Verification items for the finished model (mm, model axes). Face numbers are marked on the shaded views. A direction names the side the tool comes from. Coordinates: 2 decimals unless noted, no trailing zeros. Write each loop counter-clockwise with the first axis right and the second up, starting at its lowest first coordinate (ties: lowest second). Pieces come first, ordered by that corner, then holes. Notation, with made-up numbers: (84.5, -33.75) -> (118.5, -33.75) arc R22 ccw to (118.5, -25.75) -> close; hole circle Ø8 at (17, 35.5). An arc over 180 degrees is marked (long way). Answer in a Markdown table with one row per item.
```python
from build123d import *

# Parameters (mm, degrees)
SKETCH1_R           = 9
BOSS_EXTRUDE1_DEPTH = 4.8
SKETCH2_R           = 5
BOSS_EXTRUDE2_DEPTH = 3.5
SKETCH3_R           = 2.75
CUT_EXTRUDE1_DEPTH  = 6.8
CHAMFER1_SIZE       = 2
CHAMFER2_SIZE       = 0.6
CHAMFER2_SIZE_2     = 0.889536581
SKETCH4_R           = 1.25
CUT_EXTRUDE2_DEPTH  = 16.081910128
CIRPATTERN1_COUNT   = 7
FILLET1_R           = 1
SKETCH5_R           = 2
CUT_EXTRUDE3_DEPTH  = 16.081910248
CHAMFER3_SIZE       = 0.6
FILLET2_R           = 0.4


with BuildPart() as part:
    # Sketch1 → Boss-Extrude1 (new body)
    with BuildSketch(Plane(origin=(0, 0, 0), x_dir=(1, 0, 0), z_dir=(0, 1, 0))):
        with Locations(Location((0, 0, 0), (0, 0, 270))):
            Circle(SKETCH1_R)
    extrude(amount=BOSS_EXTRUDE1_DEPTH)

    # Sketch2 → Boss-Extrude2 (add)
    with BuildSketch(Plane(origin=(0, 4.8, 0), x_dir=(1, 0, 0), z_dir=(0, 1, 0))):
        with Locations(Location((0, 0, 0), (0, 0, 270))):
            Circle(SKETCH2_R)
    extrude(amount=BOSS_EXTRUDE2_DEPTH)

    # Sketch3 → Cut-Extrude1 (cut)
    with BuildSketch(Plane(origin=(0, 8.3, 0), x_dir=(1, 0, 0), z_dir=(0, 1, 0))):
        with Locations(Location((0, 0, 0), (0, 0, 270))):
            Circle(SKETCH3_R)
    extrude(amount=-CUT_EXTRUDE1_DEPTH, mode=Mode.SUBTRACT)

    # Chamfer1
    chamfer1_edges = [part.edges().sort_by_distance(p)[0] for p in [
        (0, 8.3, -5),
    ]]
    chamfer(chamfer1_edges, length=CHAMFER1_SIZE)

    # Chamfer2
    # the kernel refuses this chamfer: 0.889536581, 0.6 mm, written as the material it takes off along each edge
    with BuildSketch(Plane(origin=(0, 8.3, 0), x_dir=(0, 0, 1), z_dir=(-1, 0, 0))) as chamfer2_piece_1:
        Polygon((2.75 + CHAMFER2_SIZE, 0), (2.75, -CHAMFER2_SIZE_2), (2.75, 0), align=None)
    revolve(axis=Axis((0, 8.3, 0), (0, 1, 0)), mode=Mode.SUBTRACT)

    # Sketch4 → Cut-Extrude2 (cut, through all)
    with BuildSketch(Plane.XZ):
        with Locations((0, 9.5)):
            Circle(SKETCH4_R)
    cut_extrude2 = extrude(amount=-CUT_EXTRUDE2_DEPTH, mode=Mode.SUBTRACT)

    # CirPattern1: Cut-Extrude2 ×7 about axis
    cirpattern1_axis = Axis((0, 0, 0), (0, 1, 0))
    for i in range(1, CIRPATTERN1_COUNT):
        add(cut_extrude2.rotate(cirpattern1_axis, i * 360 / CIRPATTERN1_COUNT), mode=Mode.SUBTRACT)

    # Fillet1
    fillet1_edges = [part.edges().sort_by_distance(p)[0] for p in [
        (0, 1.5, -2.75),
        (-1.112946158, 2.4, 8.930921053),
        (1.112946158, 2.4, 8.930921053),
        (6.288564667, 2.4, 6.438474543),
        (7.676385826, 2.4, 4.698201853),
        (8.954658034, 2.4, -0.902274619),
        (8.459350397, 2.4, -3.072359168),
        (4.877711261, 2.4, -7.563592589),
        (2.87225158, 2.4, -8.529371071),
        (-2.87225158, 2.4, -8.529371071),
        (-4.877711261, 2.4, -7.563592589),
        (-8.459350397, 2.4, -3.072359168),
        (-8.954658034, 2.4, -0.902274619),
        (-7.676385826, 2.4, 4.698201853),
        (-6.288564667, 2.4, 6.438474543),
    ]]
    fillet(fillet1_edges, radius=FILLET1_R)

    # Sketch5 → Cut-Extrude3 (cut, through all)
    with BuildSketch(Plane.XZ):
        with Locations(Location((0, 0, 0), (0, 0, 270))):
            Circle(SKETCH5_R)
    extrude(amount=-CUT_EXTRUDE3_DEPTH, mode=Mode.SUBTRACT)

    # Chamfer3
    chamfer3_edges = [part.edges().sort_by_distance(p)[0] for p in [
        (-7.674626305, 0, 4.512162546),
        (-6.106798223, 0, 6.478156776),
        (-1.257300502, 0, 8.813551793),
        (1.257300502, 0, 8.813551793),
        (0, 4.8, 8.25),
        (6.45010973, 4.8, 5.143790865),
        (8.77435121, 4.8, 2.002688406),
        (8.043155276, 4.8, -1.835797705),
        (7.036483342, 4.8, -5.611408217),
        (3.579540848, 4.8, -7.43299316),
        (0, 4.8, -9),
        (-3.579540848, 4.8, -7.43299316),
        (-7.036483342, 4.8, -5.611408217),
        (-8.043155276, 4.8, -1.835797705),
        (-8.77435121, 4.8, 2.002688406),
        (-6.45010973, 4.8, 5.143790865),
        (-3.904953652, 4.8, 8.108719811),
        (6.106798223, 4.8, 6.478156776),
        (7.674626305, 4.8, 4.512162546),
        (8.87235333, 4.8, -0.735422423),
        (8.312801966, 4.8, -3.18697713),
        (4.956845417, 4.8, -7.395213538),
        (2.691268197, 4.8, -8.486258024),
        (-2.691268197, 4.8, -8.486258024),
        (-4.956845417, 4.8, -7.395213538),
        (-8.312801966, 4.8, -3.18697713),
        (-8.87235333, 4.8, -0.735422423),
        (-7.674626305, 4.8, 4.512162546),
        (-6.106798223, 4.8, 6.478156776),
        (-1.257300502, 4.8, 8.813551793),
        (1.257300502, 4.8, 8.813551793),
        (0, 0, 2),
        (3.904953652, 0, 8.108719811),
        (3.904953652, 4.8, 8.108719811),
        (8.77435121, 0, 2.002688406),
        (6.45010973, 0, 5.143790865),
        (0, 0, 8.25),
        (-3.904953652, 0, 8.108719811),
        (-6.45010973, 0, 5.143790865),
        (-8.77435121, 0, 2.002688406),
        (-8.043155276, 0, -1.835797705),
        (-7.036483342, 0, -5.611408217),
        (-3.579540848, 0, -7.43299316),
        (0, 0, -9),
        (3.579540848, 0, -7.43299316),
        (7.036483342, 0, -5.611408217),
        (8.043155276, 0, -1.835797705),
        (6.106798223, 0, 6.478156776),
        (7.674626305, 0, 4.512162546),
        (8.87235333, 0, -0.735422423),
        (8.312801966, 0, -3.18697713),
        (4.956845417, 0, -7.395213538),
        (2.691268197, 0, -8.486258024),
        (-2.691268197, 0, -8.486258024),
        (-4.956845417, 0, -7.395213538),
        (-8.312801966, 0, -3.18697713),
        (-8.87235333, 0, -0.735422423),
    ]]
    chamfer(chamfer3_edges, length=CHAMFER3_SIZE)

    # Fillet2
    fillet2_edges = [part.edges().sort_by_distance(p)[0] for p in [
        (0, 6.3, -5),
        (0, 7.410463419, -2.75),
        (0, 4.8, -5),
    ]]
    fillet(fillet2_edges, radius=FILLET2_R)


solid = part.part
```
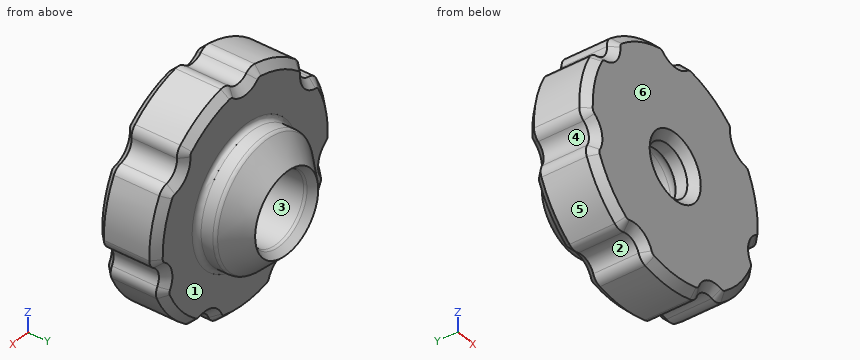
1. Sectioned sample at A-A, the plane y = 7.75. Record the cut outline in (x, z).
Findings below:
| item | result |
|---|---|
| outline | circle Ø7.1 at (0, 0); hole circle Ø5.96 at (0, 0) |
2. Material ranges on probe 1 along X at (y, z) = (5.4, 0); probe 2 along Y at (x, z) = (-7, -4); probe 3 along Z at (x, y) = (0, 1.2), recorded low to high. Write a range as from..to.
Findings below:
| item | result |
|---|---|
| probe 1 | x = -5..-2.75, 2.75..5 |
| probe 2 | y = 0..4.8 |
| probe 3 | z = -9..-2, 2..8.25 |
3. Access from +Z, -Z, +X, -X, +Y, -Y to the whole of each face (thin tool, end or side, straight path). Record for the marked faces 1 and 2.
Findings below:
| item | result |
|---|---|
| face 1 | +Y |
| face 2 | -Z, +Y, -Y |
4. Release check for a two-part mould opening along Z. For the marked faces 3, 4, 5 and 6 record: released by +Z, released by -Z, zero draft, split by the parting line, or undercut.
Findings below:
| item | result |
|---|---|
| face 3 | undercut |
| face 4 | undercut |
| face 5 | released by -Z |
| face 6 | zero draft |
5. Go/stop test with a flat-tipped pin: pin 1 (1 mm diameter, centred on x = -4, y = 4, fed in from +Z). Record where the tip stops, or that it passes through.
Findings below:
| item | result |
|---|---|
| pin 1 | stops at z = 8.29 |
